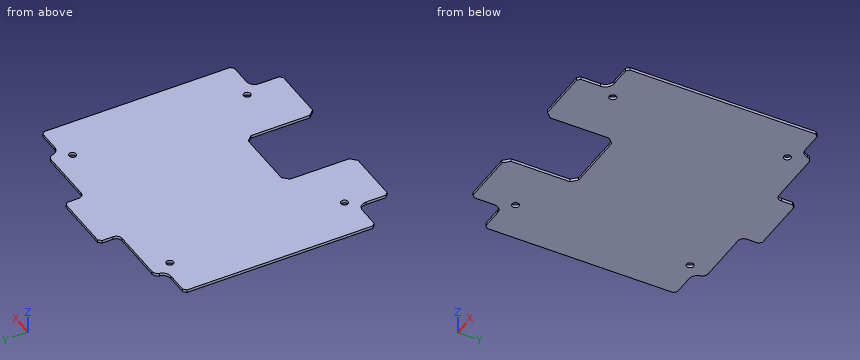
from build123d import *

# Parameters (mm, degrees)
SKETCH_1_W          = 68
SKETCH_1_H          = 68
SKETCH_1_R          = 1.25
SKETCH_1_H_2        = 11
SKETCH_1_W_2        = 11.5
EXTRUDE_2_DEPTH     = 1
FILLET_1_R          = 3
SKETCH_3_W          = 25
SKETCH_3_H          = 25
CUT_EXTRUDE_1_DEPTH = 2
CHAMFER_1_SIZE      = 2
SKETCH_5_W          = 23
SKETCH_5_H          = 7
CUT_EXTRUDE_2_DEPTH = 2
FILLET_2_R          = 2
CHAMFER_2_SIZE      = 1


with BuildPart() as part:
    # ｽｹｯﾁ1 → ﾎﾞｽ - 押し出し2 (new body)
    with BuildSketch(Plane.XY):
        Rectangle(SKETCH_1_W, SKETCH_1_H)
        with Locations((-31, -31)):
            Circle(SKETCH_1_R, mode=Mode.SUBTRACT)
        with Locations((31, -31)):
            Circle(SKETCH_1_R, mode=Mode.SUBTRACT)
        with Locations((-31, 31)):
            Circle(SKETCH_1_R, mode=Mode.SUBTRACT)
        with Locations((31, 31)):
            Circle(SKETCH_1_R, mode=Mode.SUBTRACT)
        with Locations((0, 39.5)):
            Rectangle(SKETCH_1_W, SKETCH_1_H_2)
        with Locations((-39.75, 0)):
            Rectangle(SKETCH_1_W_2, SKETCH_1_H)
        with Locations((39.75, 0)):
            Rectangle(SKETCH_1_W_2, SKETCH_1_H)
        with Locations((0, -39.5)):
            Rectangle(SKETCH_1_W, SKETCH_1_H_2)
    extrude(amount=EXTRUDE_2_DEPTH)

    # ﾌｨﾚｯﾄ1
    fillet_1_edges = [part.edges().sort_by_distance(p)[0] for p in [
        (-34, -34, 0.5),
        (-34, 34, 0.5),
        (34, 34, 0.5),
        (34, -34, 0.5),
    ]]
    fillet(fillet_1_edges, radius=FILLET_1_R)

    # ｽｹｯﾁ3 → ｶｯﾄ - 押し出し1 (cut, through all)
    with BuildSketch(Plane.XY.offset(1)):
        with Locations((0, -32.5)):
            Rectangle(SKETCH_3_W, SKETCH_3_H)
    extrude(amount=-CUT_EXTRUDE_1_DEPTH, mode=Mode.SUBTRACT)

    # 面取り1
    chamfer_1_edges = [part.edges().sort_by_distance(p)[0] for p in [
        (-12.5, -45, 0.5),
        (-12.5, -20, 0.5),
        (12.5, -20, 0.5),
        (12.5, -45, 0.5),
    ]]
    chamfer(chamfer_1_edges, length=CHAMFER_1_SIZE)

    # ｽｹｯﾁ5 → ｶｯﾄ - 押し出し2 (cut, through all)
    with BuildSketch(Plane.XY.offset(1)):
        with Locations((-22.5, 41.5)):
            Rectangle(SKETCH_5_W, SKETCH_5_H)
        with Locations((22.5, 41.5)):
            Rectangle(SKETCH_5_W, SKETCH_5_H)
    extrude(amount=-CUT_EXTRUDE_2_DEPTH, mode=Mode.SUBTRACT)

    # ﾌｨﾚｯﾄ2
    fillet_2_edges = [part.edges().sort_by_distance(p)[0] for p in [
        (11, 38, 0.5),
        (34, 38, 0.5),
        (-11, 38, 0.5),
        (-34, 38, 0.5),
    ]]
    fillet(fillet_2_edges, radius=FILLET_2_R)

    # 面取り2
    chamfer_2_edges = [part.edges().sort_by_distance(p)[0] for p in [
        (-11, 45, 0.5),
        (11, 45, 0.5),
        (34, -45, 0.5),
        (-34, -45, 0.5),
        (-45.5, -34, 0.5),
        (-45.5, 34, 0.5),
        (45.5, 34, 0.5),
        (45.5, -34, 0.5),
    ]]
    chamfer(chamfer_2_edges, length=CHAMFER_2_SIZE)


solid = part.part
Design review of the part built by this model. Coordinates are the model's own, in mm. Coordinates: 2 decimals unless noted, no trailing zeros. Write each loop counter-clockwise with the first axis right and the second up, starting at its lowest first coordinate (ties: lowest second). Pieces come first, ordered by that corner, then holes. Notation, with made-up numbers: (89.25, 72) -> (130.25, 72) arc R24 cw to (130.25, 108) -> close; hole circle Ø8 at (38.25, -25.5). An arc over 180 degrees is marked (long way). Write each question's results on one line, items separated by ' | '. Start each with the question number.
(1) For line 1 along Y through (x, z) = (-31, 0.4); line 2 along X through (y, z) = (-22, 0.75); line 3 along X through (y, z) = (-41, 0.7), list the stretches that pass through material, from the lowest coordinate up. Write a range as from..to.
(2) Clearance check with a flat-ended pin moving along its axis: P1, Ø2, axis at x = -11.5, y = 3, coming from the -Z side. State where the tip first meets the part, or that it passes through.
(3) Take a section at A-A on y = 31. Write out the cut boundary in (x, z).
(4) Take a section at C-C on z = 0.45. Give the number of separate pieces and of enclosed holes in the cut face, and give its area (3 significant figures).
(5) Take a section at D-D on x = -5. Write out the cut boundary in (y, z), and give its area (3 significant figures).
(6) Take a section at B-B on x = 31. Write out the cut boundary in (y, z).
Results found:
1) line 1: y = -45..-32.25, -29.75..29.75, 32.25..38 | line 2: x = -45.5..-12.5, 12.5..45.5 | line 3: x = -34..-12.5, 12.5..34
2) P1: stops at z = 0
3) outline: (-45.5, 0) -> (-32.25, 0) -> (-32.25, 1) -> (-45.5, 1) -> close; (-29.75, 0) -> (29.75, 0) -> (29.75, 1) -> (-29.75, 1) -> close; (32.25, 0) -> (45.5, 0) -> (45.5, 1) -> (32.25, 1) -> close
4) separate pieces: 1 | enclosed holes: 4 | area: 6,720 mm2
5) outline: (-20, 0) -> (45, 0) -> (45, 1) -> (-20, 1) -> close | area: 65.0 mm2
6) outline: (-45, 0) -> (-32.25, 0) -> (-32.25, 1) -> (-45, 1) -> close; (-29.75, 0) -> (29.75, 0) -> (29.75, 1) -> (-29.75, 1) -> close; (32.25, 0) -> (38, 0) -> (38, 1) -> (32.25, 1) -> close
